```python
from build123d import *

# Parameters (mm, degrees)
SKETCH_1_R      = 2
SKETCH_1_R_2    = 1.5
SKETCH_1_W      = 65
SKETCH_1_H      = 65
EXTRUDE_1_DEPTH = 4


with BuildPart() as part:
    # 草图1 → 凸台-拉伸1 (new body)
    with BuildSketch(Plane(origin=(0, 0, 0), x_dir=(1, 0, 0), z_dir=(0, 1, 0))):
        Polygon((119.192286341, -98.145825623), (119.192286341, -6.391560818), (47.5, 35), (47.5, 115), (-47.5, 115), (-47.5, 35), (-119.192286341, -6.391560818), (-119.192286341, -98.145825623), align=None)
        with Locations(Location((0, 19, 0), (0, 0, 270))):
            Circle(SKETCH_1_R, mode=Mode.SUBTRACT)
        with Locations(Location((25.980762114, 15, 0), (0, 0, 270))):
            Circle(SKETCH_1_R_2, mode=Mode.SUBTRACT)
        with Locations(Location((16.454482672, -9.5, 0), (0, 0, 270))):
            Circle(SKETCH_1_R, mode=Mode.SUBTRACT)
        with Locations(Location((0, -30, 0), (0, 0, 270))):
            Circle(SKETCH_1_R_2, mode=Mode.SUBTRACT)
        with Locations(Location((-16.454482672, -9.5, 0), (0, 0, 270))):
            Circle(SKETCH_1_R, mode=Mode.SUBTRACT)
        with Locations(Location((-25.980762114, 15, 0), (0, 0, 270))):
            Circle(SKETCH_1_R_2, mode=Mode.SUBTRACT)
        with Locations(Location((0, 102.5, 0), (0, 0, 270))):
            Circle(SKETCH_1_R, mode=Mode.SUBTRACT)
        with Locations(Location((-106.692286341, -85.645825623, 0), (0, 0, 270))):
            Circle(SKETCH_1_R, mode=Mode.SUBTRACT)
        with Locations(Location((106.692286341, -85.645825623, 0), (0, 0, 270))):
            Circle(SKETCH_1_R, mode=Mode.SUBTRACT)
        with Locations(Location((-43.5, 102.5, 0), (0, 0, 270))):
            Circle(SKETCH_1_R, mode=Mode.SUBTRACT)
        with Locations(Location((43.5, 102.5, 0), (0, 0, 270))):
            Circle(SKETCH_1_R, mode=Mode.SUBTRACT)
        with Locations(Location((-17.428761251, 10.0625, 0), (0, 0, 270))):
            Circle(SKETCH_1_R, mode=Mode.SUBTRACT)
        with Locations(Location((17.428761251, 10.0625, 0), (0, 0, 270))):
            Circle(SKETCH_1_R, mode=Mode.SUBTRACT)
        with Locations(Location((0, -20.125, 0), (0, 0, 270))):
            Circle(SKETCH_1_R, mode=Mode.SUBTRACT)
        with Locations((0, 57.5)):
            Rectangle(SKETCH_1_W, SKETCH_1_H, mode=Mode.SUBTRACT)
        Polygon((37.900635095, 15.645825623), (5.400635095, -40.645825623), (61.692286341, -73.145825623), (94.192286341, -16.854174377), align=None, mode=Mode.SUBTRACT)
        Polygon((-5.400635095, -40.645825623), (-37.900635095, 15.645825623), (-94.192286341, -16.854174377), (-61.692286341, -73.145825623), align=None, mode=Mode.SUBTRACT)
    extrude(amount=EXTRUDE_1_DEPTH)


solid = part.part
```
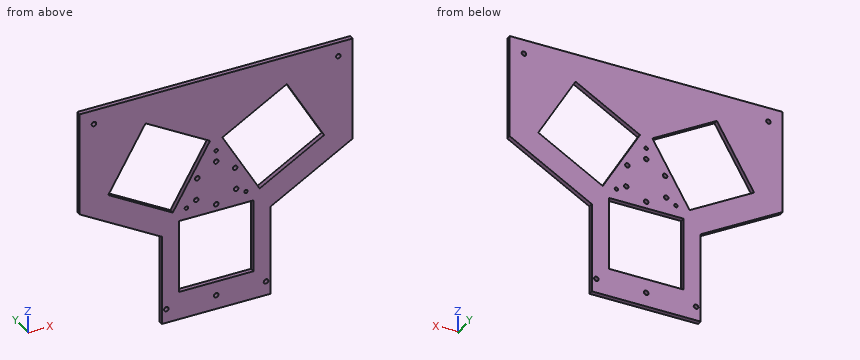
Build history of the part. All positions in model axes, mm. Give positions to 0.01 mm unless a question says otherwise; leave off trailing zeros. Loops run counter-clockwise (first coordinate to the right, second up) from the corner with the lowest first, then second, coordinate; pieces in that order, holes last.
Item 1: Slice it at A-A, the plane z = -64.5. List the corners of the cut face in (x, y).
Answers follow:
outline: (-47.5, 0) - (-32.5, 0) - (-32.5, 4) - (-47.5, 4) - close; (32.5, 0) - (47.5, 0) - (47.5, 4) - (32.5, 4) - close
Item 2: Flat gauge pins, fed straight in: pin 1 (1.2 mm diameter, centred on y = 3, z = -53.5, fed in from -X); pin 2 (1.2 mm diameter, centred on y = 1, z = -54.5, fed in from +X). Where does each tip first touch, or does it go through?
Answers follow:
pin 1: stops at x = -47.5
pin 2: stops at x = 47.5
Item 3: Drill centre lines: line 1 (X direction, y = 2.15, z = -11); line 2 (X direction, y = 2.9, z = -38); line 3 (X direction, y = 3.7, z = 32.5). Where is each one in solid material? Low to high.
Answers follow:
line 1: x = -89.07 to -45.95, -35.22 to -19.2, -15.66 to 15.66, 19.2 to 35.22, 45.95 to 89.07
line 2: x = -47.5 to -32.5, 32.5 to 47.5
line 3: x = -119.19 to -85.16, -10.1 to 10.1, 85.16 to 119.19
Item 4: Slice it at D-D, the plane y = 1.45. Give the number of separate pieces and of enclosed holes in the cut face, and give its area (3 significant figures).
Answers follow:
separate pieces: 1
enclosed holes: 17
area: 23,500 mm2
Item 5: Slice it at C-C, the plane z = 63.5. List the corners of the cut face in (x, y), and give its area (3 significant figures).
Answers follow:
outline: (-119.19, 0) - (-67.26, 0) - (-67.26, 4) - (-119.19, 4) - close; (-44.99, 0) - (44.99, 0) - (44.99, 4) - (-44.99, 4) - close; (67.26, 0) - (119.19, 0) - (119.19, 4) - (67.26, 4) - close
area: 775 mm2
Item 6: Slice it at B-B, the plane x = 55.5. List the corners of the cut face in (y, z), and give its area (3 significant figures).
Answers follow:
outline: (0, -30.38) - (4, -30.38) - (4, -5.48) - (0, -5.48) - close; (0, 69.57) - (4, 69.57) - (4, 98.15) - (0, 98.15) - close
area: 214 mm2
